```python
from build123d import *

# Parameters (mm, degrees)
F1_DEPTH = 38.1
F2_T     = -2.54
F3_T     = 2.54


with BuildPart() as f1:
    # F0 (on Right) → F1 (new body, symmetric)
    with BuildSketch(Plane.YZ):
        with BuildLine():
            Line((277.3325320094, 76.2), (-112.5278806646, 76.2))
            ThreePointArc((-112.5278806646, 76.2), (-90.5951741668, 37.8398160871), (-113.4139305449, 0))
            Line((-113.4139305449, 0), (326.9511687087, 0))
            Line((326.9511687087, 0), (277.3325320094, 76.2))
        make_face()
    extrude(amount=F1_DEPTH, both=True)

    # F2
    f2_openings = [f1.faces().sort_by_distance(p)[0] for p in [
        (0, -90.595174, 37.839816),
    ]]
    offset(amount=F2_T, openings=f2_openings)

    # F3
    f3_openings = [f1.faces().sort_by_distance(p)[0] for p in [
        (0, 302.14185, 38.1),
    ]]
    offset(amount=F3_T, openings=f3_openings, kind=Kind.INTERSECTION)


solid = f1.part
```
Input: part model. Units: mm. Frame: model coordinates. A direction names the side the tool comes from. Give positions to 0.01 mm unless a question says otherwise; leave off trailing zeros. Order: outer loops, then holes, each group sorted by start corner. A loop starts at its lowest first (then second) coordinate and runs counter-clockwise, first axis right, second up. Notation, with made-up numbers: M 49,0 L 55,0 A22 cw 55,17 Z; hole C -12,7.25 d7. An arc over 180 degrees is marked long. Return JSON: item names as keys, results as strings.
Item 1: Cut plane C-C (y = 281.5). Return loops of the section in (x, z).
Solutions:
{"outline": "M -40.64,-2.54 L 40.64,-2.54 L 40.64,69.8 L 38.1,69.8 L 38.1,0 L -38.1,0 L -38.1,69.8 L -40.64,69.8 Z; M -35.56,2.54 L 35.56,2.54 L 35.56,65.15 L -35.56,65.15 Z; hole M -33.02,5.08 L 33.02,5.08 L 33.02,60.49 L -33.02,60.49 Z"}
Item 2: Cut plane D-D (z = 50). Return loops of the section in (x, y).
Solutions:
{"outline": "M -40.64,-94.82 L -33.02,-94.82 L -33.02,288.33 L 33.02,288.33 L 33.02,-94.82 L 40.64,-94.82 L 40.64,294.39 L 38.1,294.39 L 38.1,-92.18 L 35.56,-92.18 L 35.56,291.36 L -35.56,291.36 L -35.56,-92.18 L -38.1,-92.18 L -38.1,294.39 L -40.64,294.39 Z"}
Item 3: Access query for faces 4 (the flat face through (0, 86, 73.66)), 5 (the flat face through (1, 77, 78.74)), 6 (the flat face through (-33.02, 101, 39)). Directions: +Z, -Z, +X, -X, +Y, -Y. A direction counts if a zero-diameter tool reaches every point of the face in a straight line with its end or side. Return the directions, or none.
Solutions:
{"face 4": "+Y", "face 5": "+Z, +X, -X, +Y, -Y", "face 6": "-Y"}
Item 4: Pull-direction query (X, two-part tool) for faces 1 (the flat face through (-40.64, 96, 39)), 2 (the flat face through (0, 85, 71.12)), 3 (the flat face through (40.64, 96, 39)); classes: +X half, -X half, draft (parallel to the pull), parting line (faces both ways), or undercut.
Solutions:
{"face 1": "-X half", "face 2": "undercut", "face 3": "+X half"}
Item 5: Ray query, probe 1 along Z at (x, y) = (-4.5, 214.5); probe 2 along X at (y, z) = (-88.5, 52); probe 3 along X at (y, z) = (92, 2). Return the intervals inside material, ascending.
Solutions:
{"probe 1": "-2.54 to 0, 2.54 to 5.08, 71.12 to 73.66, 76.2 to 78.74", "probe 2": "-40.64 to -38.1, -35.56 to -33.02, 33.02 to 35.56, 38.1 to 40.64", "probe 3": "-40.64 to -38.1, 38.1 to 40.64"}
Item 6: Cut plane B-B (x = 20.5). Return loops of the section in (y, z), then the cut area to 3 significant figures.
Solutions:
{"outline": "M -130.16,-2.54 L 328.61,-2.54 L 326.95,0 L -113.41,0 A43.63 ccw -109.3,2.54 L 322.27,2.54 L 275.96,73.66 L -108.6,73.66 A43.63 ccw -112.53,76.2 L 277.33,76.2 L 275.68,78.74 L -126.69,78.74 A41.09 cw -109.44,71.12 L 274.58,71.12 L 317.58,5.08 L -110.11,5.08 A41.09 cw Z", "area": "4,470 mm^2"}
Item 7: First-contact query: P1, Ø1.5, axis at x = -12.5, z = 47.5, coming from the +Y side; P2, Ø5, axis at x = -11.5, z = 28, coming from the -Y side. Flat tips, straight axial feed; report the tip coordinate or a pass-through.
Solutions:
{"P1": "y = 293.48", "P2": "y = 301.03"}
Item 8: Cut plane A-A (y = -8). Return loops of the section in (x, z).
Solutions:
{"outline": "M -40.64,-2.54 L 40.64,-2.54 L 40.64,78.74 L -40.64,78.74 Z; M -35.56,2.54 L 35.56,2.54 L 35.56,73.66 L -35.56,73.66 Z; hole M -38.1,0 L 38.1,0 L 38.1,76.2 L -38.1,76.2 Z; hole M -33.02,5.08 L 33.02,5.08 L 33.02,71.12 L -33.02,71.12 Z"}
